```python
from build123d import *

# Parameters (mm, degrees)
SKETCH_1_W          = 25
SKETCH_1_H          = 20
EXTRUDE_1_DEPTH     = 13
SHELL_7_T           = -1.5
SKETCH_3_R          = 1.5
CUT_EXTRUDE_1_DEPTH = 5
SKETCH_4_W          = 15
SKETCH_4_H          = 10
CUT_EXTRUDE_2_DEPTH = 2
SKETCH_6_W          = 12.730573974
SKETCH_6_H          = 22.360557323
CUT_EXTRUDE_5_DEPTH = 38.5
EXTRUDE_START       = -1.5
EXTRUDE_4_OUTLINE_R = 3
EXTRUDE_4_DEPTH     = 1.5
EXTRUDE_5_DEPTH     = 11.5
SKETCH_12_R         = 1.475
CUT_EXTRUDE_6_DEPTH = 1.5
SKETCH_14_R         = 1.475
CUT_EXTRUDE_7_DEPTH = 27
FILLET_2_R          = 0.5
FILLET_3_R          = 0.5
FILLET_4_R          = 0.5
FILLET_5_R          = 0.5
FILLET_6_R          = 0.5
FILLET_7_R          = 0.5


with BuildPart() as part:
    # 草图1 → 凸台-拉伸1 (new body)
    with BuildSketch(Plane.XY):
        Rectangle(SKETCH_1_W, SKETCH_1_H)
    extrude(amount=EXTRUDE_1_DEPTH)

    # 抽壳7
    shell_7_openings = [part.faces().sort_by_distance(p)[0] for p in [
        (0, 0, 13),
    ]]
    offset(amount=SHELL_7_T, openings=shell_7_openings, kind=Kind.INTERSECTION)

    # 草图3 → 切除-拉伸1 (cut)
    with BuildSketch(Plane.XY.offset(1.5)):
        with Locations((-10.25, 0)):
            Circle(SKETCH_3_R)
        with Locations((10.25, 0)):
            Circle(SKETCH_3_R)
    extrude(amount=-CUT_EXTRUDE_1_DEPTH, mode=Mode.SUBTRACT)

    # 草图4 → 切除-拉伸2 (cut)
    with BuildSketch(Plane.XY.offset(1.5)):
        Rectangle(SKETCH_4_W, SKETCH_4_H)
    extrude(amount=-CUT_EXTRUDE_2_DEPTH, mode=Mode.SUBTRACT)

    # 草图6 → 切除-拉伸5 (cut, symmetric)
    with BuildSketch(Plane(origin=(-11, 0, 0), x_dir=(0, 0, -1), z_dir=(1, 0, 0))):
        with Locations((-7.865286987, 2.680278662)):
            Rectangle(SKETCH_6_W, SKETCH_6_H)
    extrude(amount=CUT_EXTRUDE_5_DEPTH, both=True, mode=Mode.SUBTRACT)

    # 凸台-拉伸4: read off the stored shape, not the designer's step
    # 凸台-拉伸4 outline → 凸台-拉伸4 (add)
    with BuildSketch(Plane(origin=(0, -8.5, 0), x_dir=(1, 0, 0), z_dir=(0, 1, 0)).offset(EXTRUDE_START)):
        with BuildLine():
            Line((15.5, -1.5), (-15.5, -1.5))
            ThreePointArc((-15.5, -1.5), (-21.25, -7.25), (-15.5, -13))
            Line((-15.5, -13), (15.5, -13))
            ThreePointArc((15.5, -13), (21.25, -7.25), (15.5, -1.5))
        make_face()
        with Locations((-15.5, -7.25)):
            Circle(EXTRUDE_4_OUTLINE_R, mode=Mode.SUBTRACT)
        with Locations((15.5, -7.25)):
            Circle(EXTRUDE_4_OUTLINE_R, mode=Mode.SUBTRACT)
    extrude(amount=EXTRUDE_4_DEPTH)

    # 草图11 → 凸台-拉伸5 (add)
    with BuildSketch(Plane.XY.offset(1.5)):
        Polygon((-11, 8.5), (11, 8.5), (11, 3), (12.5, 3), (12.5, 10), (-12.5, 10), (-12.5, 3), (-11, 3), align=None)
    extrude(amount=EXTRUDE_5_DEPTH)

    # 草图12 → 切除-拉伸6 (cut)
    with BuildSketch(Plane(origin=(0, 10, 0), x_dir=(1, 0, 0), z_dir=(0, 1, 0))):
        with Locations(Location((-8, -6.5, 0), (0, 0, 270))):
            Circle(SKETCH_12_R)
        with Locations(Location((8, -6.5, 0), (0, 0, 90))):
            Circle(SKETCH_12_R)
    extrude(amount=-CUT_EXTRUDE_6_DEPTH, mode=Mode.SUBTRACT)

    # 草图14 → 切除-拉伸7 (cut)
    with BuildSketch(Plane.ZY.offset(12.5)):
        with Locations(Location((6.5, 5.5, 0), (0, 0, 270))):
            Circle(SKETCH_14_R)
    extrude(amount=-CUT_EXTRUDE_7_DEPTH, mode=Mode.SUBTRACT)

    # 圆角2
    fillet_2_edges = [part.edges().sort_by_distance(p)[0] for p in [
        (-12.5, 0, 0),
    ]]
    fillet(fillet_2_edges, radius=FILLET_2_R)

    # 圆角3
    fillet_3_edges = [part.edges().sort_by_distance(p)[0] for p in [
        (12.5, 0, 0),
    ]]
    fillet(fillet_3_edges, radius=FILLET_3_R)

    # 圆角4
    fillet_4_edges = [part.edges().sort_by_distance(p)[0] for p in [
        (12.5, 3, 7.25),
    ]]
    fillet(fillet_4_edges, radius=FILLET_4_R)

    # 圆角5
    fillet_5_edges = [part.edges().sort_by_distance(p)[0] for p in [
        (11, 3, 7.25),
    ]]
    fillet(fillet_5_edges, radius=FILLET_5_R)

    # 圆角6
    fillet_6_edges = [part.edges().sort_by_distance(p)[0] for p in [
        (-12.5, 3, 7.25),
    ]]
    fillet(fillet_6_edges, radius=FILLET_6_R)

    # 圆角7
    fillet_7_edges = [part.edges().sort_by_distance(p)[0] for p in [
        (-11, 3, 7.25),
    ]]
    fillet(fillet_7_edges, radius=FILLET_7_R)


solid = part.part
```
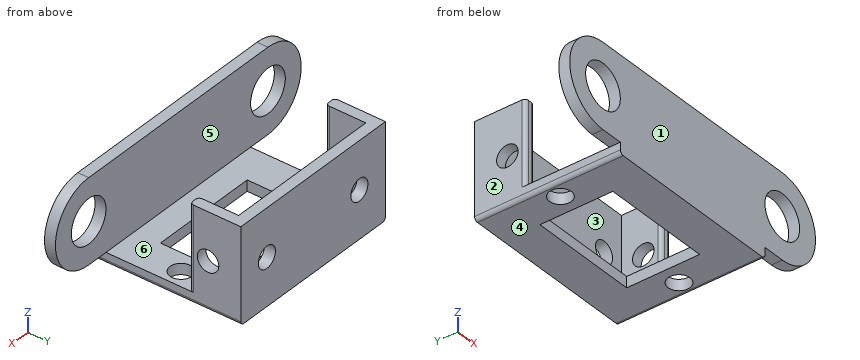
Could you check a few things on this model? Use its own coordinates, in mm. Face numbers are marked on the shaded views. A direction names the side the tool comes from. Give positions to 0.01 mm unless a question says otherwise; leave off trailing zeros. Write each loop counter-clockwise with the first axis right and the second up, starting at its lowest first coordinate (ties: lowest second). Pieces come first, ordered by that corner, then holes. Notation, with made-up numbers: (-34, 10) -> (6, 10) arc R11 ccw to (6, 16) -> close; hole circle Ø11 at (-17.5, 50). An arc over 180 degrees is marked (long way). Write each question's results on one line, items separated by ' | '.
1. I want a section at B-B, the plane y = -4.5. Write out the boundary of the cut face in (x, z), then the cut area to 3 significant figures.
Check sheet entries:
outline: (-12.5, 0.5) arc R0.5 ccw to (-12, 0) -> (-7.5, 0) -> (-7.5, 1.5) -> (-12.5, 1.5) -> close; (7.5, 0) -> (12, 0) arc R0.5 ccw to (12.5, 0.5) -> (12.5, 1.5) -> (7.5, 1.5) -> close | area: 14.9 mm²
2. I want a section at A-A, the plane x = -8. Write out the boundary of the cut face in (y, z) (3 decimals), then the cut area to 3 significant figures.
Check sheet entries:
outline: (-10, 0) -> (10, 0) -> (10, 5.025) -> (8.5, 5.025) -> (8.5, 1.5) -> (-8.5, 1.5) -> (-8.5, 13) -> (-10, 13) -> close; (8.5, 7.975) -> (10, 7.975) -> (10, 13) -> (8.5, 13) -> close | area: 60.1 mm²
3. I want a section at D-D, the plane z = 3.5. Write out the boundary of the cut face in (x, y), then the cut area to 3 significant figures.
Check sheet entries:
outline: (-19.86, -10) -> (19.86, -10) -> (19.86, -8.5) -> (-19.86, -8.5) -> close; (-12.5, 3.5) arc R0.5 ccw to (-12, 3) -> (-11.5, 3) arc R0.5 ccw to (-11, 3.5) -> (-11, 8.5) -> (11, 8.5) -> (11, 3.5) arc R0.5 ccw to (11.5, 3) -> (12, 3) arc R0.5 ccw to (12.5, 3.5) -> (12.5, 10) -> (-12.5, 10) -> close | area: 113 mm²
4. If we mould it in two halves opening along Y, with no side actions, what happens to the marked faces 1, 2 and 3? For each: released by +Y, released by -Y, zero draft, split by the parting line, or undercut.
Check sheet entries:
face 1: released by -Y | face 2: zero draft | face 3: undercut
5. Will these pins go through, and if not, where does the flat tip stop? pin 1 Ø10 at (x, y) = (5.5, 2.5) entering from +Z; pin 2 Ø1.5 at (y, z) = (7, 9.5) entering from -X; pin 3 Ø1.8 at (x, z) = (8, 6.5) entering from +Y; pin 4 Ø2.5 at (x, y) = (10.25, 0) entering from -Z.
Check sheet entries:
pin 1: stops at z = 1.5 | pin 2: stops at x = -12.5 | pin 3: stops at y = -8.5 | pin 4: passes through
6. On a 3-axis mill with a long thin cutter (end or side, diameter ignored), from which of +Z, -Z, +X, -X, +Y, -Y can I reach the whole of each face in a straight line? I mean the marked faces 4, 5 and 6. Say none if no direction works.
Check sheet entries:
face 4: -Z, +X, -X, +Y, -Y | face 5: +Z, +X, -X | face 6: +Z
7. I want a section at C-C, the plane y = 5.5. Write out the boundary of the cut face in (x, z) (3 decimals), then the cut area to 3 significant figures.
Check sheet entries:
outline: (-12.5, 0.5) arc R0.5 ccw to (-12, 0) -> (12, 0) arc R0.5 ccw to (12.5, 0.5) -> (12.5, 5.025) -> (11, 5.025) -> (11, 1.5) -> (-11, 1.5) -> (-11, 5.025) -> (-12.5, 5.025) -> close; (-12.5, 7.975) -> (-11, 7.975) -> (-11, 13) -> (-12.5, 13) -> close; (11, 7.975) -> (12.5, 7.975) -> (12.5, 13) -> (11, 13) -> close | area: 63.0 mm²
8. I need wall thicknesses on L1, parallel to X at y = 0, z = 0.85; L2, parallel to X at y = -9.15, z = 7.25; L3, parallel to Y at x = -1.5, z = 10.5. Which ranges of each line are inside material? Lowest first, please.
Check sheet entries:
L1: x = -12.5 to -11.75, -8.75 to -7.5, 7.5 to 8.75, 11.75 to 12.5 | L2: x = -21.25 to -18.5, -12.5 to 12.5, 18.5 to 21.25 | L3: y = -10 to -8.5, 8.5 to 10
